Check sheet for the modelled part. Datum: model origin and axes. Units: mm. A direction names the side the tool comes from. Give positions to 0.01 mm unless a question says otherwise; leave off trailing zeros. Order: outer loops, then holes, each group sorted by start corner. A loop starts at its lowest first (then second) coordinate and runs counter-clockwise, first axis right, second up.
from build123d import *

# Parameters (mm, degrees)
SKETCH1_R           = 42.5
BOSS_EXTRUDE1_DEPTH = 5
SKETCH2_R           = 27.5
BOSS_EXTRUDE2_DEPTH = 10
SKETCH3_R           = 7.5
CUT_EXTRUDE1_DEPTH  = 8
SKETCH4_R           = 1.5
CUT_EXTRUDE2_DEPTH  = 16
SKETCH5_R           = 2
CUT_EXTRUDE3_DEPTH  = 6


with BuildPart() as part:
    # Sketch1 → Boss-Extrude1 (new body)
    with BuildSketch(Plane.XY):
        Circle(SKETCH1_R)
    extrude(amount=BOSS_EXTRUDE1_DEPTH)

    # Sketch2 → Boss-Extrude2 (add)
    with BuildSketch(Plane.XY.offset(5)):
        Circle(SKETCH2_R)
    extrude(amount=BOSS_EXTRUDE2_DEPTH)

    # Sketch3 → Cut-Extrude1 (cut)
    with BuildSketch(Plane.XY.offset(15)):
        Circle(SKETCH3_R)
    extrude(amount=-CUT_EXTRUDE1_DEPTH, mode=Mode.SUBTRACT)

    # Sketch4 → Cut-Extrude2 (cut, through all)
    with BuildSketch(Plane.XY.offset(15)):
        with Locations((0, 10)):
            Circle(SKETCH4_R)
        with Locations((10, 0)):
            Circle(SKETCH4_R)
        with Locations((0, -10)):
            Circle(SKETCH4_R)
        with Locations((-10, 0)):
            Circle(SKETCH4_R)
    extrude(amount=-CUT_EXTRUDE2_DEPTH, mode=Mode.SUBTRACT)

    # Sketch5 → Cut-Extrude3 (cut, through all)
    with BuildSketch(Plane.XY.offset(5)):
        with Locations((0, 32.5)):
            Circle(SKETCH5_R)
        with Locations((22.980970389, 22.980970389)):
            Circle(SKETCH5_R)
        with Locations((32.5, 0)):
            Circle(SKETCH5_R)
        with Locations((22.980970389, -22.980970389)):
            Circle(SKETCH5_R)
        with Locations((0, -32.5)):
            Circle(SKETCH5_R)
        with Locations((-22.980970389, -22.980970389)):
            Circle(SKETCH5_R)
        with Locations((-32.5, 0)):
            Circle(SKETCH5_R)
        with Locations((-22.980970389, 22.980970389)):
            Circle(SKETCH5_R)
    extrude(amount=-CUT_EXTRUDE3_DEPTH, mode=Mode.SUBTRACT)


solid = part.part
1) Material ranges on L1, parallel to Y at x = 0, z = 6.5; L2, parallel to Y at x = 0.5, z = 0.5; L3, parallel to Z at x = 18, y = -30, recorded low to high.
Recorded:
L1: y = -27.5 to -11.5, -8.5 to 8.5, 11.5 to 27.5
L2: y = -42.5 to -34.44, -30.56 to -11.41, -8.59 to 8.59, 11.41 to 30.56, 34.44 to 42.5
L3: z = 0 to 5
2) Section check B-B, the plane z = 2.75. State how many separate pieces and enclosed holes the cut face has, then the cut area to 3 significant figures.
Recorded:
separate pieces: 1
enclosed holes: 12
area: 5,550 mm2
3) Depth check by flat-ended pin: pin 1 Ø6.5 at (x, y) = (32.5, 0) entering from +Z; pin 2 Ø3.5 at (x, y) = (-22.98, 22.98) entering from -Z; pin 3 Ø1 at (y, z) = (22, 2.5) entering from +X; pin 4 Ø2 at (x, z) = (-22, 10.5) entering from -Y. Enter the tip coordinate at first touch or a pass-through.
Recorded:
pin 1: stops at z = 5
pin 2: passes through
pin 3: stops at x = 36.66
pin 4: stops at y = -17.76
4) Section check D-D, the plane x = 32. Record the cut outline in (y, z), then the cut area to 3 significant figures.
Recorded:
outline: (-27.97, 0) - (-1.94, 0) - (-1.94, 5) - (-27.97, 5) - close; (1.94, 0) - (27.97, 0) - (27.97, 5) - (1.94, 5) - close
area: 260 mm2
5) Section check C-C, the plane y = 10. Record the cut outline in (x, z), then the cut area to 3 significant figures.
Recorded:
outline: (-41.31, 0) - (-1.5, 0) - (-1.5, 15) - (-25.62, 15) - (-25.62, 5) - (-41.31, 5) - close; (1.5, 0) - (41.31, 0) - (41.31, 5) - (25.62, 5) - (25.62, 15) - (1.5, 15) - close
area: 880 mm2
6) Set-up check for faces 4 (the face through (0, 0, 7)), 5 (the face through (-0.434, -34.452, 2.535)): record each of +Z, -Z, +X, -X, +Y, -Y from which the full face is reachable in a straight line by a thin tool's end or side.
Recorded:
face 4: +Z
face 5: +Z, -Z
7) Draft check along Y on faces 1 (the face through (-5.961, -26.846, 9.93)), 2 (the face through (24.89, 23.58, 2.54)), 3 (the face through (-1, 1, 0)). Enter one of: +Y half, -Y half, draft (parallel to the pull), parting line (faces both ways), or undercut.
Recorded:
face 1: parting line
face 2: undercut
face 3: draft
8) Section check A-A, the plane x = 0. Record the cut outline in (y, z).
Recorded:
outline: (-42.5, 0) - (-34.5, 0) - (-34.5, 5) - (-42.5, 5) - close; (-30.5, 0) - (-11.5, 0) - (-11.5, 15) - (-27.5, 15) - (-27.5, 5) - (-30.5, 5) - close; (-8.5, 0) - (8.5, 0) - (8.5, 15) - (7.5, 15) - (7.5, 7) - (-7.5, 7) - (-7.5, 15) - (-8.5, 15) - close; (11.5, 0) - (30.5, 0) - (30.5, 5) - (27.5, 5) - (27.5, 15) - (11.5, 15) - close; (34.5, 0) - (42.5, 0) - (42.5, 5) - (34.5, 5) - close
